Design review of the part built by this model. Coordinates are the model's own, in mm. A direction names the side the tool comes from. Give positions to 0.01 mm unless a question says otherwise; leave off trailing zeros. Loops run counter-clockwise (first coordinate to the right, second up) from the corner with the lowest first, then second, coordinate; pieces in that order, holes last. Notation, with made-up numbers: (12, 21) - (57, 21) arc R24 cw to (57, 46) - close; hole circle Ø6 at (85, 62.25). An arc over 180 degrees is marked (long way). One line per item, written item: value. Start each with the question number.
```python
from build123d import *

# Parameters (mm, degrees)
SKETCH_2_W               = 32
SKETCH_2_H               = 32
SKETCH_2_W_2             = 26
SKETCH_2_H_2             = 26
EXTRUDE_1_DEPTH          = 26
SKETCH_3_W               = 62
SKETCH_3_H               = 72
EXTRUDE_2_DEPTH          = 7.5
FILLET_1_R               = 2
FILLET_2_R               = 2
CUT_EXTRUDE_1_DEPTH      = 66.88626564
CUT_EXTRUDE_1_DEPTH_BACK = 66.88626564
SKETCH_5_R               = 1.1
SKETCH_5_R_2             = 8.5
FILLET_3_R               = 2
SKETCH_7_R               = 0.85
CUT_EXTRUDE_2_DEPTH      = 70.189955918
FILLET_4_R               = 10
CUT_EXTRUDE_3_DEPTH      = 66.88626564


with BuildPart() as part:
    # ｽｹｯﾁ2 → ﾎﾞｽ - 押し出し1 (new body)
    with BuildSketch(Plane.XY):
        with Locations((0, 16)):
            Rectangle(SKETCH_2_W, SKETCH_2_H)
        with Locations((0, 16)):
            Rectangle(SKETCH_2_W_2, SKETCH_2_H_2, mode=Mode.SUBTRACT)
    extrude(amount=EXTRUDE_1_DEPTH)

    # ｽｹｯﾁ3 → ﾎﾞｽ - 押し出し2 (add)
    with BuildSketch(Plane(origin=(0, 0, 0), x_dir=(-1, 0, 0), z_dir=(0, 0, -1))):
        with Locations((0, 16)):
            Rectangle(SKETCH_3_W, SKETCH_3_H)
    extrude(amount=EXTRUDE_2_DEPTH)

    # ﾌｨﾚｯﾄ1
    fillet_1_edges = [part.edges().sort_by_distance(p)[0] for p in [
        (0, 32, 0),
        (16, 16, 0),
        (0, 0, 0),
        (-16, 16, 0),
    ]]
    fillet(fillet_1_edges, radius=FILLET_1_R)

    # ﾌｨﾚｯﾄ2
    fillet_2_edges = [part.edges().sort_by_distance(p)[0] for p in [
        (31, 16, 0),
        (0, -20, 0),
        (-31, 16, 0),
        (0, 52, 0),
    ]]
    fillet(fillet_2_edges, radius=FILLET_2_R)

    # ｽｹｯﾁ5 → ｶｯﾄ - 押し出し1 (cut, two sides: drawn at the far end of the back side and taken through both)
    with BuildSketch(Plane.XZ.offset(-CUT_EXTRUDE_1_DEPTH_BACK)):
        with Locations(Location((10.5, 23.5, 0), (0, 0, 270))):
            Circle(SKETCH_5_R)
        with Locations(Location((-10.5, 23.5, 0), (0, 0, 270))):
            Circle(SKETCH_5_R)
        with Locations(Location((-10.5, 2.5, 0), (0, 0, 332.964308211))):
            Circle(SKETCH_5_R)
        with Locations(Location((10.5, 2.5, 0), (0, 0, 332.964308211))):
            Circle(SKETCH_5_R)
        with Locations((0, 23.5)):
            Circle(SKETCH_5_R_2)
    extrude(amount=CUT_EXTRUDE_1_DEPTH + CUT_EXTRUDE_1_DEPTH_BACK, mode=Mode.SUBTRACT)

    # ﾌｨﾚｯﾄ3
    fillet_3_edges = [part.edges().sort_by_distance(p)[0] for p in [
        (8.124038405, 1.5, 26),
        (-8.124038405, 1.5, 26),
        (-8.124038405, 30.5, 26),
        (8.124038405, 30.5, 26),
    ]]
    fillet(fillet_3_edges, radius=FILLET_3_R)

    # ｽｹｯﾁ7 → ｶｯﾄ - 押し出し2 (cut, through all)
    with BuildSketch(Plane(origin=(0, 0, -7.5), x_dir=(-1, 0, 0), z_dir=(0, 0, -1))):
        with Locations((-23.5, -10)):
            Circle(SKETCH_7_R)
        with Locations((-23.5, 42)):
            Circle(SKETCH_7_R)
        with Locations((23.5, 42)):
            Circle(SKETCH_7_R)
        with Locations((23.5, -10)):
            Circle(SKETCH_7_R)
    extrude(amount=-CUT_EXTRUDE_2_DEPTH, mode=Mode.SUBTRACT)

    # ﾌｨﾚｯﾄ4
    # the kernel refuses this fillet: 10 mm, written as the material it takes off along each edge
    with BuildSketch(Plane(origin=(21, -10, 0), x_dir=(0, -1, 0), z_dir=(-1, 0, 0))) as fillet_4_piece_1:
        with BuildLine():
            CenterArc((8, -2), 2, 0, 90)
            Line((10, -2), (10, 0))
            Line((10, 0), (8, 0))
        make_face()
    revolve(axis=Axis((21, -10, 0), (0, 0, 1)), revolution_arc=90, mode=Mode.SUBTRACT)
    with BuildSketch(Plane(origin=(21, 42, 0), x_dir=(1, 0, 0), z_dir=(0, -1, 0))) as fillet_4_piece_2:
        with BuildLine():
            CenterArc((8, -2), 2, 0, 90)
            Line((10, -2), (10, 0))
            Line((10, 0), (8, 0))
        make_face()
    revolve(axis=Axis((21, 42, 0), (0, 0, 1)), revolution_arc=90, mode=Mode.SUBTRACT)
    with BuildSketch(Plane(origin=(-21, -10, 0), x_dir=(-1, 0, 0), z_dir=(0, 1, 0))) as fillet_4_piece_3:
        with BuildLine():
            CenterArc((8, -2), 2, 0, 90)
            Line((10, -2), (10, 0))
            Line((10, 0), (8, 0))
        make_face()
    revolve(axis=Axis((-21, -10, 0), (0, 0, 1)), revolution_arc=90, mode=Mode.SUBTRACT)
    with BuildSketch(Plane(origin=(-21, 42, 0), x_dir=(0, 1, 0), z_dir=(1, 0, 0))) as fillet_4_piece_4:
        with BuildLine():
            CenterArc((8, -2), 2, 0, 90)
            Line((10, -2), (10, 0))
            Line((10, 0), (8, 0))
        make_face()
    revolve(axis=Axis((-21, 42, 0), (0, 0, 1)), revolution_arc=90, mode=Mode.SUBTRACT)
    with BuildSketch(Plane(origin=(31, 52, 0), x_dir=(0, -1, 0), z_dir=(0, 0, -1)), Plane(origin=(-31, 52, 0), x_dir=(1, 0, 0), z_dir=(0, 0, -1))) as fillet_4_piece_5:
        with BuildLine():
            CenterArc((FILLET_4_R, FILLET_4_R), FILLET_4_R, 180, 90)
            Line((0, FILLET_4_R), (0, 0))
            Line((0, 0), (FILLET_4_R, 0))
        make_face()
    extrude(amount=32.5, mode=Mode.SUBTRACT)
    with BuildSketch(Plane(origin=(31, -20, 0), x_dir=(0, 1, 0), z_dir=(0, 0, -1)), Plane(origin=(-31, -20, 0), x_dir=(1, 0, 0), z_dir=(0, 0, -1))) as fillet_4_piece_6:
        with BuildLine():
            CenterArc((FILLET_4_R, -FILLET_4_R), FILLET_4_R, 90, 90)
            Line((0, -FILLET_4_R), (0, 0))
            Line((0, 0), (FILLET_4_R, 0))
        make_face()
    extrude(amount=32.5, mode=Mode.SUBTRACT)

    # ｽｹｯﾁ8 → ｶｯﾄ - 押し出し3 (cut, through all)
    with BuildSketch(Plane.XY):
        with BuildLine():
            Line((-17.5, 47), (17.5, 47))
            ThreePointArc((17.5, 47), (18.560660172, 46.560660172), (19, 45.5))
            Line((19, 45.5), (19, 38.5))
            ThreePointArc((19, 38.5), (18.560660172, 37.439339828), (17.5, 37))
            Line((17.5, 37), (-17.5, 37))
            ThreePointArc((-17.5, 37), (-18.560660172, 37.439339828), (-19, 38.5))
            Line((-19, 38.5), (-19, 45.5))
            ThreePointArc((-19, 45.5), (-18.560660172, 46.560660172), (-17.5, 47))
        make_face()
        with BuildLine():
            Line((22.5, 33), (24.5, 33))
            ThreePointArc((24.5, 33), (25.560660172, 32.560660172), (26, 31.5))
            Line((26, 31.5), (26, 0.5))
            ThreePointArc((26, 0.5), (25.560660172, -0.560660172), (24.5, -1))
            Line((24.5, -1), (22.5, -1))
            ThreePointArc((22.5, -1), (21.439339828, -0.560660172), (21, 0.5))
            Line((21, 0.5), (21, 31.5))
            ThreePointArc((21, 31.5), (21.439339828, 32.560660172), (22.5, 33))
        make_face()
        with BuildLine():
            Line((-24.5, 33), (-22.5, 33))
            ThreePointArc((-22.5, 33), (-21.439339828, 32.560660172), (-21, 31.5))
            Line((-21, 31.5), (-21, 0.5))
            ThreePointArc((-21, 0.5), (-21.439339828, -0.560660172), (-22.5, -1))
            Line((-22.5, -1), (-24.5, -1))
            ThreePointArc((-24.5, -1), (-25.560660172, -0.560660172), (-26, 0.5))
            Line((-26, 0.5), (-26, 31.5))
            ThreePointArc((-26, 31.5), (-25.560660172, 32.560660172), (-24.5, 33))
        make_face()
        with BuildLine():
            Line((-17.5, -5), (17.5, -5))
            ThreePointArc((17.5, -5), (18.560660172, -5.439339828), (19, -6.5))
            Line((19, -6.5), (19, -13.5))
            ThreePointArc((19, -13.5), (18.560660172, -14.560660172), (17.5, -15))
            Line((17.5, -15), (-17.5, -15))
            ThreePointArc((-17.5, -15), (-18.560660172, -14.560660172), (-19, -13.5))
            Line((-19, -13.5), (-19, -6.5))
            ThreePointArc((-19, -6.5), (-18.560660172, -5.439339828), (-17.5, -5))
        make_face()
    extrude(amount=-CUT_EXTRUDE_3_DEPTH, mode=Mode.SUBTRACT)


solid = part.part
```
(1) Draft analysis for pull direction X (two halves, no side actions). For faces 1 (the cylindrical face through (27.99, 49.15, -4.71)), 2 (the flat face through (0, 3, 10)), 3 (the flat face through (14, 16, 26)), state which applies: pulls with the +X half, pulls with the -X half, needs draft (parallel to the pull), parting line crosses it, or undercut.
(2) Take a section at B-B on y = 14. State the section outline as (x, z) points, and give its area (3 significant figures).
(3) Take a section at A-A on x = -14. State the section outline as (y, z) points, and give its area (3 significant figures).
(4) Take a section at D-D on x = 0. State the section outline as (y, z) points.
(5) To check wall thickness, follow L1, parallel to Y at x = 4.5, z = -3.5; L2, parallel to Z at x = -10.5, y = 30.85; L3, parallel to X at y = 31.2, z = 2.5. State the ranges of each line that lie inside material, in increasing order. Write a range as from..to.
(6) For pin 1 Ø2 at (x, z) = (10.5, 2.5) entering from -Y; pin 2 Ø2 at (y, z) = (3.5, 13.5) entering from -X; pin 3 Ø2.5 at (x, z) = (-10.5, 23.5) entering from -Y; pin 4 Ø5 at (x, y) = (5, 13.5) entering from +Z, all flat-tipped, find the tip position at first contact; note any pin that passes through.
(7) Take a section at C-C on y = 35. State the section outline as (x, z) points, and give its area (3 significant figures).
(8) Machinability: for faces 4 (the flat face through (0, 32, 11)), 5 (the flat face through (-24, 33, -4)), 6 (the flat face through (0, 29, 10)), 7 (the flat face through (-16, 16, 14)), 8 (the flat face through (0, 0, 11)), which of the approach directions +Z, -Z, +X, -X, +Y, -Y give a long, thin tool a straight path to every point of the face, cutting with its end or side? Answer none if there is none.
Here are the results:
1. face 1: pulls with the +X half
1. face 2: undercut
1. face 3: needs draft
2. outline: (-31, -7.5) - (-26, -7.5) - (-26, 0) - (-29, 0) arc R2 ccw to (-31, -2) - close; (-21, -7.5) - (21, -7.5) - (21, 0) - (18, 0) arc R2 cw to (16, 2) - (16, 26) - (13, 26) - (13, 0) - (-13, 0) - (-13, 26) - (-16, 26) - (-16, 2) arc R2 cw to (-18, 0) - (-21, 0) - close; (26, -7.5) - (31, -7.5) - (31, -2) arc R2 ccw to (29, 0) - (26, 0) - close
2. area: 546 mm²
3. outline: (-20, -7.5) - (-15, -7.5) - (-15, 0) - (-18, 0) arc R2 ccw to (-20, -2) - close; (-5, -7.5) - (37, -7.5) - (37, 0) - (34, 0) arc R2 cw to (32, 2) - (32, 26) - (0, 26) - (0, 2) arc R2 cw to (-2, 0) - (-5, 0) - close; (47, -7.5) - (52, -7.5) - (52, -2) arc R2 ccw to (50, 0) - (47, 0) - close
3. area: 1,220 mm²
4. outline: (-20, -7.5) - (-15, -7.5) - (-15, 0) - (-18, 0) arc R2 ccw to (-20, -2) - close; (-5, -7.5) - (37, -7.5) - (37, 0) - (34, 0) arc R2 cw to (32, 2) - (32, 15) - (29, 15) - (29, 0) - (3, 0) - (3, 15) - (0, 15) - (0, 2) arc R2 cw to (-2, 0) - (-5, 0) - close; (47, -7.5) - (52, -7.5) - (52, -2) arc R2 ccw to (50, 0) - (47, 0) - close
5. L1: -20..-15, -5..37, 47..52
5. L2: -7.5..1.4, 3.6..22.4, 24.6..26
5. L3: -16..-11.6, -9.4..9.4, 11.6..16
6. pin 1: through
6. pin 2: x = -16
6. pin 3: y = 0
6. pin 4: z = 0
7. outline: (-31, -7.5) - (31, -7.5) - (31, -2) arc R2 ccw to (29, 0) - (-29, 0) arc R2 ccw to (-31, -2) - close
7. area: 463 mm²
8. face 4: +Z, +X, -X, +Y
8. face 5: +Z, -Z
8. face 6: +Z
8. face 7: +Z, -X, +Y, -Y
8. face 8: +Z, +X, -X, -Y
